The model under review builds one solid part; all positions refer to its coordinate system, in mm. Face numbers are marked on the shaded views. A direction names the side the tool comes from. Give positions to 0.01 mm unless a question says otherwise; leave off trailing zeros. Order: outer loops, then holes, each group sorted by start corner. A loop starts at its lowest first (then second) coordinate and runs counter-clockwise, first axis right, second up.
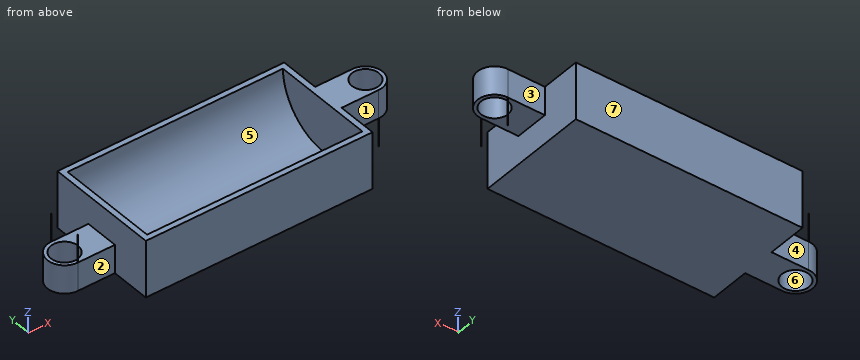
Solid Edge part; units mm, degrees
sketch "Sketch1" plane through (0, 0, 0) normal (0, 0, 1) x (1, 0, 0)
  line L0 (6.55, 10) -> (6.55, 2.999963)
  line L1 (0.014946, 2.999963) -> (6.55, 2.999963)
  line L2 (6.55, -2.999963) -> (0.014946, -2.999963)
  line L3 (6.55, -2.999963) -> (6.55, -10)
  line L4 (6.55, -10) -> (46.55, -10)
  line L5 (46.55, -10) -> (46.55, -2.999963)
  line L6 (53.085054, -2.999963) -> (46.55, -2.999963)
  line L7 (46.55, 2.999963) -> (53.085054, 2.999963)
  line L8 (46.55, 2.999963) -> (46.55, 10)
  line L9 (46.55, 10) -> (6.55, 10)
  arc A0 (0.0149, -2.999963) -> (0.0149, 2.999963) centre (0, 0) cw
  arc A1 (53.0851, 2.999963) -> (53.0851, -2.999963) centre (53.1, 0) cw
  circle A2 centre (0, 0) radius 2.38
  circle A3 centre (53.1, 0) radius 2.38
extrude "Protrusion1" add sketch "Sketch1" along normal blind 10
sketch "Sketch2" plane through (45.55, -6.499981, 5) normal (1, 0, 0) x (0, 1, 0)
  circle A0 centre (6.499981, 5) radius 9
extrude "ExtrudedCutout_1" cut sketch "Sketch2" against normal blind 38
sketch "Sketch3" plane through (26.55, 0, 0) normal (0, 0, -1) x (1, 0, 0)
  line L0 (29.55, -2.999963) -> (29.55, 2.999963)
  line L1 (29.55, 2.999963) -> (20, 2.999963)
  line L2 (20, 2.999963) -> (20, -2.999963)
  line L3 (20, -2.999963) -> (29.55, -2.999963)
extrude "ExtrudedCutout_2" cut sketch "Sketch3" against normal blind 5
sketch "Sketch4" plane through (26.55, 0, 10) normal (0, 0, 1) x (1, 0, 0)
  line L0 (-20, -2.999963) -> (-29.835403, -2.999963)
  line L1 (-29.835403, -2.999963) -> (-29.835403, 2.999963)
  line L2 (-29.835403, 2.999963) -> (-20, 2.999963)
  line L3 (-20, 2.999963) -> (-20, -2.999963)
extrude "ExtrudedCutout_3" cut sketch "Sketch4" against normal blind 5
1. For the marked faces 1, 2, 3, 4 and 5, list the 3-axis set-ups (+Z, -Z, +X, -X, +Y, -Y) from which the entire face can be reached by the end or side of a thin tool; tool diameter is ignored.
2. Take a section at B-B (y = 0). Write out the cut boundary in (x, z).
3. Insertion check: pin 1 (3 mm diameter, centred on x = 51.5, y = -0.5, fed in from -Z); pin 2 (3 mm diameter, centred on y = 3, z = 5.5, fed in from +X); pin 3 (5.5 mm diameter, centred on x = 48.5, z = 7.5, fed in from +Y); pin 4 (1.5 mm diameter, centred on x = 25, y = -3.5, fed in from +Z). Each pin has a flat end and moves straight along its axis. Give the tip position at first contact, or say it passes through.
4. Draft analysis for pull direction X (two halves, no side actions). For the marked faces 6 and 7, state which applies: pulls with the +X half, pulls with the -X half, needs draft (parallel to the pull), parting line crosses it, or undercut.
5. Take a section at D-D (x = 27). Write out the cut boundary in (y, z).
6. Take a section at C-C (x = 1.5). Write out the cut boundary in (y, z), and give its area (3 significant figures).
7. To check wall thickness, follow line 1 (X direction, y = 0, z = 3.5); line 2 (X direction, y = 0, z = 8.55); line 3 (Y direction, x = 0, z = 3.2). State the ranges of each line that lie inside material, in increasing order.
Answer:
1. face 1: +Z, -Z, +X, -Y
1. face 2: +Z, -Z, -X, -Y
1. face 3: +Z, -Z, +X, +Y
1. face 4: +Z, -Z, -X, +Y
1. face 5: +Z
2. outline: (-3, 0) - (-2.38, 0) - (-2.38, 5) - (-3, 5) - close; (2.38, 0) - (46.55, 0) - (46.55, 5) - (50.72, 5) - (50.72, 10) - (45.55, 10) - (45.55, 1) - (7.55, 1) - (7.55, 10) - (6.55, 10) - (6.55, 5) - (2.38, 5) - close; (55.48, 5) - (56.1, 5) - (56.1, 10) - (55.48, 10) - close
3. pin 1: stops at z = 5
3. pin 2: stops at x = 55.7
3. pin 3: stops at y = 10
3. pin 4: stops at z = 2.07
4. face 6: undercut
4. face 7: needs draft
5. outline: (-10, 0) - (10, 0) - (10, 10) - (9, 10) arc R9 cw to (-9, 10) - (-10, 10) - close
6. outline: (-3, 0) - (-1.85, 0) - (-1.85, 5) - (-3, 5) - close; (1.85, 0) - (3, 0) - (3, 5) - (1.85, 5) - close
6. area: 11.5 mm2
7. line 1: x = -3 to -2.38, 2.38 to 7.55, 45.55 to 46.55
7. line 2: x = 6.55 to 7.55, 45.55 to 50.72, 55.48 to 56.1
7. line 3: y = -3 to -2.38, 2.38 to 3
